```python
from build123d import *

# Parameters (mm, degrees)
F0_R     = 28.575
F1_DEPTH = 40.2336
F2_R     = 3.302
F4_R     = 10.16
F5_DEPTH = 15.7734


with BuildPart() as f1:
    # F0 (on Top) → F1 (new body)
    with BuildSketch(Plane.XY):
        with Locations((-37.4545902014, -20.9862291813)):
            Circle(F0_R)
    extrude(amount=F1_DEPTH)

    # F2
    f2_edges = [f1.edges().sort_by_distance(p)[0] for p in [
        (-66.02959, -20.986229, 40.2336),
    ]]
    fillet(f2_edges, radius=F2_R)

    # F4 (on face) → F5 (join)
    with BuildSketch(Plane(origin=(0, 0, 0), x_dir=(1, 0, 0), z_dir=(0, 0, -1))):
        with BuildLine():
            Line((-65.3540068038, 14.8094032778), (-54.8419142609, -32.6714961972))
            ThreePointArc((-54.8419142609, -32.6714961972), (-35.9806114834, -52.0378622288), (-16.7446354188, -33.0435972896))
            Line((-16.7446354188, -33.0435972896), (-9.202451986, 16.7028530294))
            ThreePointArc((-9.202451986, 16.7028530294), (-36.4915787142, -7.5725388922), (-65.3540068038, 14.8094032778))
        make_face()
        with Locations((-35.7945565225, -32.9887708187)):
            Circle(F4_R, mode=Mode.SUBTRACT)
    extrude(amount=-F5_DEPTH)


solid = f1.part
```
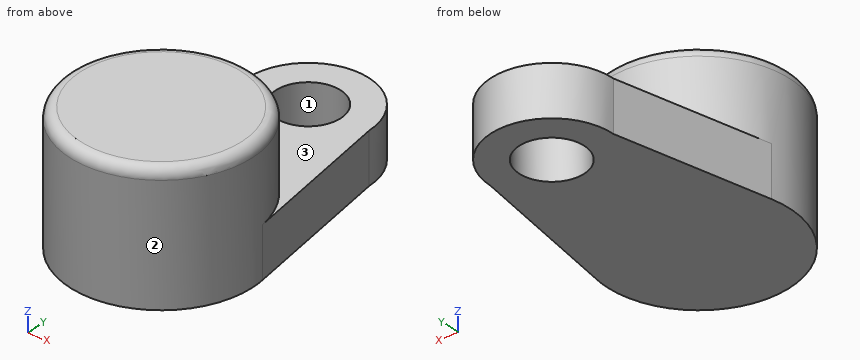
Geometry: final body of the model. Coordinates: model frame, mm. Face numbers are marked on the shaded views. Coordinates: 2 decimals unless noted, no trailing zeros. Order: outer loops, then holes, each group sorted by start corner. A loop starts at its lowest first (then second) coordinate and runs counter-clockwise, first axis right, second up. Notation, with made-up numbers: M -39,-32.5 L -11,-32.5 A28 cw -11,-9.5 Z; hole C -11,66.5 d10. An arc over 180 degrees is marked long. Answer in a Markdown table with one row per item. Add a question column.
Q1. Section query C-C on z = 38.5. Return the cut outline in (x, y), and give its area (3 significant figures).
Q2. Contact query for flat-ended pins moving along their axis: P1, Ø12, axis at x = -35.79, y = 32.99, coming from the -Z side; P2, Ø8, axis at x = -46.5, z = 18.5, coming from the -Y side; P3, Ø6, axis at y = 26.5, z = 15.5, coming from the -X side; P4, Ø6, axis at x = -17, z = 11.5, coming from the +Y side. Output: stop coordinate, or through.
Q3. Mould query, pull axis Y, two halves, no side actions, for the marked faces 1, 2 and 3. Classes: released by +Y, released by -Y, zero draft, split by the parting line, or undercut.
Q4. Line query: L1, parallel to Y at x = -35, z = 9.5; L2, parallel to Z at x = -33, y = 11; L3, parallel to Y at x = -39, z = 18. Output: solid intervals per line, ascending.
Q5. Section query B-B on y = 12. Return the cut outline in (x, z).
Completed:
| question | item | result |
|---|---|---|
| 1 | outline | C -37.45,-20.99 d56.36 |
| 1 | area | 2,490 mm2 |
| 2 | P1 | passes through |
| 2 | P2 | stops at y = -49.11 |
| 2 | P3 | stops at x = -56.87 |
| 2 | P4 | stops at y = 43.64 |
| 3 | face 1 | undercut |
| 3 | face 2 | split by the parting line |
| 3 | face 3 | zero draft |
| 4 | L1 | y = -49.46 to 22.86, 43.12 to 52.02 |
| 4 | L2 | z = 0 to 15.77 |
| 4 | L3 | y = -49.52 to 7.55 |
| 5 | outline | M -59.42,0 L -13.55,0 L -13.55,15.77 L -59.42,15.77 Z |
